from build123d import *

# Parameters (mm, degrees)
BOSS_EXTRUDE1_DEPTH = 10
SKETCH3_R           = 3.2
CUT_EXTRUDE1_DEPTH  = 2
SKETCH4_R           = 2
CUT_EXTRUDE2_DEPTH  = 2


with BuildPart() as part:
    # Sketch2 → Boss-Extrude1 (new body)
    with BuildSketch(Plane(origin=(0, 0, 0), x_dir=(0, 0, -1), z_dir=(1, 0, 0))):
        Polygon((-10.05355663, 145), (-10.05355663, 130), (0, 15.087321886), (0, 0), (-2, 0), (-2, 15), (-12.05355663, 129.912678114), (-12.05355663, 145), align=None)
    extrude(amount=BOSS_EXTRUDE1_DEPTH)

    # Sketch3 → Cut-Extrude1 (cut)
    with BuildSketch(Plane.XY.offset(2)):
        with Locations((5, 7.5)):
            Circle(SKETCH3_R)
    extrude(amount=-CUT_EXTRUDE1_DEPTH, mode=Mode.SUBTRACT)

    # Sketch4 → Cut-Extrude2 (cut)
    with BuildSketch(Plane.XY.offset(12.05355663)):
        with Locations((5, 137.5)):
            Circle(SKETCH4_R)
    extrude(amount=-CUT_EXTRUDE2_DEPTH, mode=Mode.SUBTRACT)


solid = part.part
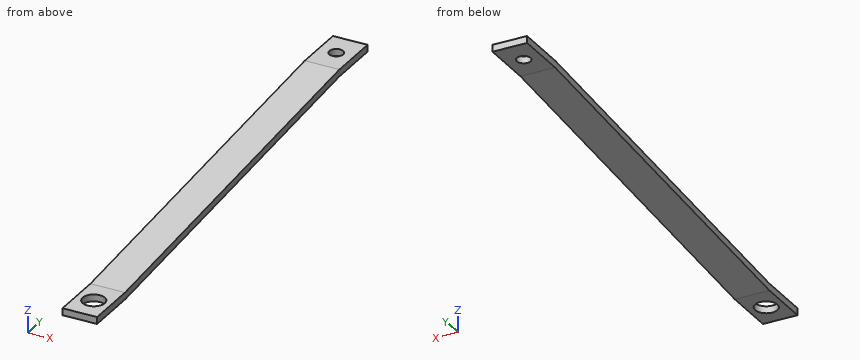
Could you check a few things on this model? Use its own coordinates, in mm. Round coordinates to 2 decimals unless told otherwise and drop trailing zeros. Write each loop counter-clockwise with the first axis right and the second up, starting at its lowest first coordinate (ties: lowest second). Pieces come first, ordered by that corner, then holes. Notation, with made-up numbers: (38, 2) -> (61, 2) arc R26 cw to (61, 37) -> close; hole circle Ø5 at (-25, 36.5). An arc over 180 degrees is marked (long way). Use a Markdown table: item, result.
1. If we section it at D-D (z = 7): List the corners of the cut face in (x, y) for me.
Answer key:
| item | result |
|---|---|
| outline | (0, 72.15) -> (10, 72.15) -> (10, 95.1) -> (0, 95.1) -> close |
2. If we section it at B-B (x = 5): List the corners of the cut face in (y, z) for me, then the cut area to 3 significant figures.
Answer key:
| item | result |
|---|---|
| outline | (0, 0) -> (4.3, 0) -> (4.3, 2) -> (0, 2) -> close; (10.7, 0) -> (15.09, 0) -> (130, 10.05) -> (135.5, 10.05) -> (135.5, 12.05) -> (129.91, 12.05) -> (15, 2) -> (10.7, 2) -> close; (139.5, 10.05) -> (145, 10.05) -> (145, 12.05) -> (139.5, 12.05) -> close |
| area | 270 mm^2 |
3. If we section it at C-C (y = 137.5): List the corners of the cut face in (x, z) for me.
Answer key:
| item | result |
|---|---|
| outline | (0, 10.05) -> (3, 10.05) -> (3, 12.05) -> (0, 12.05) -> close; (7, 10.05) -> (10, 10.05) -> (10, 12.05) -> (7, 12.05) -> close |
4. Please list where these lines run through material, in increasing order: probe 1 along X at (y, z) = (137.5, 10.7); probe 2 along Z at (x, y) = (6.75, 14.5); probe 3 along Z at (x, y) = (4, 39.5).
Answer key:
| item | result |
|---|---|
| probe 1 | x = 0 to 3, 7 to 10 |
| probe 2 | z = 0 to 2 |
| probe 3 | z = 2.14 to 4.14 |
5. For pin 1 Ø1 at (x, y) = (5, 83) entering from +Z; pin 2 Ø5 at (x, y) = (5, 136.5) entering from -Z; pin 3 Ø5 at (x, y) = (5, 7.5) entering from +Z; pin 4 Ø3 at (x, y) = (7.5, 104) entering from +Z, each with a flat end and sliding along its axis, tell me the tip position at first contact or that it passes through.
Answer key:
| item | result |
|---|---|
| pin 1 | stops at z = 7.99 |
| pin 2 | stops at z = 10.05 |
| pin 3 | passes through |
| pin 4 | stops at z = 9.92 |
6. If we section it at A-A (y = 7.5): List the corners of the cut face in (x, z) for me, then the cut area to 3 significant figures.
Answer key:
| item | result |
|---|---|
| outline | (0, 0) -> (1.8, 0) -> (1.8, 2) -> (0, 2) -> close; (8.2, 0) -> (10, 0) -> (10, 2) -> (8.2, 2) -> close |
| area | 7.20 mm^2 |
